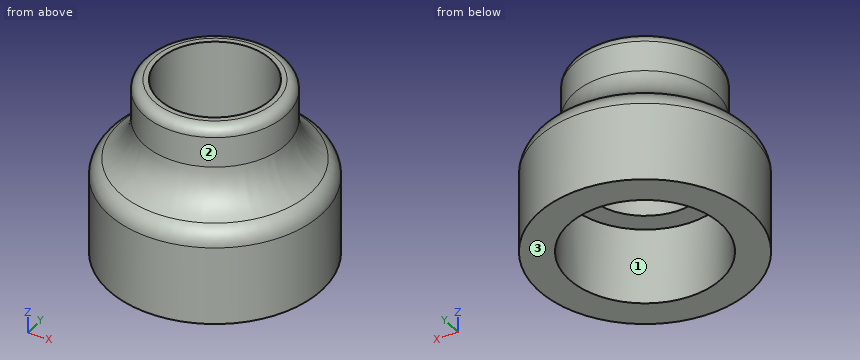
from build123d import *


with BuildPart() as f1:
    # F0 (on Front) → F1 (revolve)
    with BuildSketch(Plane.XZ):
        with BuildLine():
            Line((7.5, 7.5), (7.5, 0))
            Line((7.5, 0), (10.5, 0))
            Line((10.5, 0), (10.5, 7.733719))
            ThreePointArc((10.5, 7.733719), (10.209701, 8.771468), (9.423077, 9.507959))
            ThreePointArc((9.423077, 9.507959), (7.653173, 11.165065), (7, 13.5))
            Line((7, 13.5), (7, 16.5))
            ThreePointArc((7, 16.5), (6.707107, 17.207107), (6, 17.5))
            Line((6, 17.5), (5.500039, 17.5))
            Line((5.500039, 17.5), (5.500039, 7.5))
            Line((5.500039, 7.5), (7.5, 7.5))
        make_face()
    revolve(axis=Axis((0, 0, 9.159326), (0, 0, 1)))


solid = f1.part
Verification items for the finished model (mm, model axes). Face numbers are marked on the shaded views. Coordinates: 2 decimals unless noted, no trailing zeros. Order: outer loops, then holes, each group sorted by start corner. A loop starts at its lowest first (then second) coordinate and runs counter-clockwise, first axis right, second up. Notation, with made-up numbers: (9.25, -12.5) -> (59.25, -12.5) arc R8 cw to (59.25, 1.5) -> close; hole circle Ø7 at (-14, 31.5). An arc over 180 degrees is marked (long way). Use CSV: the item, a comma, the result in double quotes. Start each with the question number.
Q1. Section check C-C, the plane z = 5.5. Record the cut outline in (x, y), and give its area (3 significant figures).
Q2. Draft check along X on the marked faces 1, 2 and 3. Enter one of: +X half, -X half, draft (parallel to the pull), parting line (faces both ways), or undercut.
Q3. Thickness scan on line 1 along Y through (x, z) = (-0.25, 3.75); line 2 along Y through (x, z) = (0, 13.25); line 3 along X through (y, z) = (-3.5, 10.25). Record the ranges inside material, lowest first.
Q4. Section check A-A, the plane y = 0. Record the cut outline in (x, z).
Q5. Depth check by flat-ended pin: P1, Ø8, axis at x = 2, z = 8, coming from the +Y side; P2, Ø3, axis at x = 4.5, z = 6.5, coming from the +Y side; P3, Ø1.5, axis at y = 0.5, z = 12.5, coming from the -X side; P4, Ø10, axis at x = 0, y = 0, coming from the -Z side. Enter the tip coordinate at first touch or a pass-through.
Q6. Section check D-D, the plane z = 12.5. Record the cut outline in (x, y), and give its area (3 significant figures).
Returned:
1,outline,"circle Ø21 at (0, 0); hole circle Ø15 at (0, 0)"
1,area,"170 mm^2"
2,face 1,"undercut"
2,face 2,"parting line"
2,face 3,"draft"
3,line 1,"y = -10.5 to -7.5, 7.5 to 10.5"
3,line 2,"y = -7.01 to -5.5, 5.5 to 7.01"
3,line 3,"x = -7.62 to -4.24, 4.24 to 7.62"
4,outline,"(-10.5, 0) -> (-7.5, 0) -> (-7.5, 7.5) -> (-5.5, 7.5) -> (-5.5, 17.5) -> (-6, 17.5) arc R1 ccw to (-7, 16.5) -> (-7, 13.5) arc R4.5 cw to (-9.42, 9.51) arc R2 ccw to (-10.5, 7.73) -> close; (5.5, 7.5) -> (7.5, 7.5) -> (7.5, 0) -> (10.5, 0) -> (10.5, 7.73) arc R2 ccw to (9.42, 9.51) arc R4.5 cw to (7, 13.5) -> (7, 16.5) arc R1 ccw to (6, 17.5) -> (5.5, 17.5) -> close"
5,P1,"stops at y = 10.5"
5,P2,"stops at y = 10.06"
5,P3,"stops at x = -7.34"
5,P4,"passes through"
6,outline,"circle Ø14.23 at (0, 0); hole circle Ø11 at (0, 0)"
6,area,"63.9 mm^2"
